```python
from build123d import *

# Parameters (mm, degrees)
BOSS_EXTRUDE1_DEPTH = 3.175
SKETCH3_R           = 1.47
CUT_EXTRUDE5_DEPTH  = 10
CUT_EXTRUDE6_DEPTH  = 10
BOSS_EXTRUDE2_DEPTH = 3.175
SKETCH7_R           = 1.5
CUT_EXTRUDE7_DEPTH  = 10
SKETCH9_R           = 1.5
CUT_EXTRUDE9_DEPTH  = 10
CUT_EXTRUDE10_DEPTH = 10
SKETCH11_R          = 1.5
CUT_EXTRUDE11_DEPTH = 10


with BuildPart() as part:
    # Sketch1 → Boss-Extrude1 (new body)
    with BuildSketch(Plane.XY):
        Polygon((-26.794919243, 100), (26.794919243, 100), (73.205080757, 73.205080757), (100, 26.794919243), (100, -26.794919243), (73.205080757, -73.205080757), (26.794919243, -100), (-26.794919243, -100), (-73.205080757, -73.205080757), (-100, -26.794919243), (-100, 26.794919243), (-73.205080757, 73.205080757), align=None)
    extrude(amount=BOSS_EXTRUDE1_DEPTH)

    # Sketch3 → Cut-Extrude5 (cut)
    with BuildSketch(Plane(origin=(0, 0, 0), x_dir=(-1, 0, 0), z_dir=(0, 0, -1))):
        Polygon((51.443588913, -82.102909721), (53.031088913, -84.852540378), (73.205080757, -73.205080757), (84.852540378, -53.031088913), (82.102909721, -51.443588913), (70.880819443, -70.880819443), align=None)
        Polygon((-26.794919243, -100), (-3.5, -100), (-3.5, -96.825), (-25.944180557, -96.825), (-45.381411087, -85.602909721), (-46.968911087, -88.352540378), align=None)
        Polygon((-73.205080757, -73.205080757), (-53.031088913, -84.852540378), (-51.443588913, -82.102909721), (-70.880819443, -70.880819443), (-82.102909721, -51.443588913), (-84.852540378, -53.031088913), align=None)
        with Locations((-49.20625, -85.22772505)):
            Circle(SKETCH3_R)
        Polygon((-100, -26.794919243), (-88.352540378, -46.968911087), (-85.602909721, -45.381411087), (-96.825, -25.944180557), (-96.825, -3.5), (-100, -3.5), align=None)
        Polygon((-100, 26.794919243), (-100, 3.5), (-96.825, 3.5), (-96.825, 25.944180557), (-85.602909721, 45.381411087), (-88.352540378, 46.968911087), align=None)
        Polygon((-26.794919243, 100), (-46.968911087, 88.352540378), (-45.381411087, 85.602909721), (-25.944180557, 96.825), (-3.5, 96.825), (-3.5, 100), align=None)
        Polygon((26.794919243, 100), (3.5, 100), (3.5, 96.825), (25.944180557, 96.825), (45.381411087, 85.602909721), (46.968911087, 88.352540378), align=None)
        Polygon((73.205080757, 73.205080757), (53.031088913, 84.852540378), (51.443588913, 82.102909721), (70.880819443, 70.880819443), (82.102909721, 51.443588913), (84.852540378, 53.031088913), align=None)
        with Locations((-85.22772505, 49.20625)):
            Circle(SKETCH3_R)
        with Locations((-49.20625, 85.22772505)):
            Circle(SKETCH3_R)
        with Locations((0, 98.4125)):
            Circle(SKETCH3_R)
        with Locations((49.20625, 85.22772505)):
            Circle(SKETCH3_R)
        with Locations((85.22772505, 49.20625)):
            Circle(SKETCH3_R)
        with Locations((98.4125, 0)):
            Circle(SKETCH3_R)
        Polygon((96.825, -3.5), (96.825, -25.944180557), (85.602909721, -45.381411087), (88.352540378, -46.968911087), (100, -26.794919243), (100, -3.5), align=None)
        with Locations((85.22772505, -49.20625)):
            Circle(SKETCH3_R)
        Polygon((45.381411087, -85.602909721), (25.944180557, -96.825), (3.5, -96.825), (3.5, -100), (26.794919243, -100), (46.968911087, -88.352540378), align=None)
        with Locations((0, -98.4125)):
            Circle(SKETCH3_R)
        with Locations((49.20625, -85.22772505)):
            Circle(SKETCH3_R)
        with Locations((-85.22772505, -49.20625)):
            Circle(SKETCH3_R)
        with Locations((-98.4125, 0)):
            Circle(SKETCH3_R)
        Polygon((-82.102909721, 51.443588913), (-70.880819443, 70.880819443), (-51.443588913, 82.102909721), (-53.031088913, 84.852540378), (-73.205080757, 73.205080757), (-84.852540378, 53.031088913), align=None)
        Polygon((100, 26.794919243), (88.352540378, 46.968911087), (85.602909721, 45.381411087), (96.825, 25.944180557), (96.825, 3.5), (100, 3.5), align=None)
    extrude(amount=-CUT_EXTRUDE5_DEPTH, mode=Mode.SUBTRACT)

    # Sketch4 → Cut-Extrude6 (cut)
    with BuildSketch(Plane.XY.offset(3.175)):
        Polygon((27.531680557, 99.574630657), (25.944180557, 96.825), (96.825, -25.944180557), (100, -25.944180557), (100, 27.816263625), (73.190593106, 73.213445206), align=None)
    extrude(amount=-CUT_EXTRUDE6_DEPTH, mode=Mode.SUBTRACT)

    # Sketch5 → Boss-Extrude2 (add)
    with BuildSketch(Plane.XY.offset(3.175)):
        Polygon((96.825, -25.944180557), (143.278603525, 0.875819943), (72.397784082, 123.6450005), (25.944180557, 96.825), align=None)
    extrude(amount=-BOSS_EXTRUDE2_DEPTH)

    # Sketch7 → Cut-Extrude7 (cut)
    with BuildSketch(Plane(origin=(0, 0, 0), x_dir=(-1, 0, 0), z_dir=(0, 0, -1))):
        with Locations((-119.051801763, -10.8021295)):
            Circle(SKETCH7_R)
        with Locations((-50.17098232, 108.502949442)):
            Circle(SKETCH7_R)
    extrude(amount=-CUT_EXTRUDE7_DEPTH, mode=Mode.SUBTRACT)

    # Sketch9 → Cut-Extrude9 (cut)
    with BuildSketch(Plane(origin=(0, 0, 0), x_dir=(-1, 0, 0), z_dir=(0, 0, -1))):
        with Locations((73.306739868, -14.507270856)):
            Circle(SKETCH9_R)
        with Locations((21.70291705, -2.187552088)):
            Circle(SKETCH9_R)
        with Locations((7.673469234, -26.303617148)):
            Circle(SKETCH9_R)
    extrude(amount=-CUT_EXTRUDE9_DEPTH, mode=Mode.SUBTRACT)

    # Sketch10 → Cut-Extrude10 (cut)
    with BuildSketch(Plane.XY.offset(3.175)):
        Polygon((27.153871113, -53.276548933), (85.191651102, -19.768396257), (26.553283992, 81.796259373), (-31.484495997, 48.288106697), align=None)
    extrude(amount=-CUT_EXTRUDE10_DEPTH, mode=Mode.SUBTRACT)

    # Sketch11 → Cut-Extrude11 (cut)
    with BuildSketch(Plane.XY.offset(3.175)):
        with Locations((64.18037908, -50.392061509)):
            Circle(SKETCH11_R)
        with Locations((-9.45962092, 77.156159961)):
            Circle(SKETCH11_R)
    extrude(amount=-CUT_EXTRUDE11_DEPTH, mode=Mode.SUBTRACT)


solid = part.part
```
Input: part model. Units: mm. Frame: model coordinates. A direction names the side the tool comes from. Coordinates: 2 decimals unless noted, no trailing zeros. Loops run counter-clockwise (first coordinate to the right, second up) from the corner with the lowest first, then second, coordinate; pieces in that order, holes last.
Q1. Line query: line 1 along Y through (x, z) = (-52.5, 1.7); line 2 along X through (y, z) = (-84, 2.65); line 3 along Y through (x, z) = (52.5, 2.05). Output: solid intervals per line, ascending.
Results are:
line 1: y = -85.16 to -83.93, -81.49 to 81.49, 83.93 to 85.16
line 2: x = -52.54 to -50.01, -48.4 to 48.4, 50.01 to 52.54
line 3: y = -85.16 to -83.93, -81.49 to -38.64, 36.86 to 112.16
Q2. Section D-D, the plane y = -66. Return the cut outline in (x, z) (3 decimals), and give its area (3 significant figures).
Results are:
outline: (-73.699, 0) - (73.699, 0) - (73.699, 3.175) - (-73.699, 3.175) - close
area: 468 mm2
Q3. Contact query for flat-ended pins moving along their axis: pin 1 (1.6 mm diameter, centred on y = -17, z = 2, fed in from -X) (3 decimals); pin 2 (1 mm diameter, centred on x = -21.5, z = 2.5, fed in from -Y) (3 decimals); pin 3 (1 mm diameter, centred on y = 35, z = 1.5, fed in from -X); pin 4 (4.5 mm diameter, centred on x = 85.23, y = -49.21, fed in from +Z) (3 decimals). Output: stop coordinate, or through.
Results are:
pin 1: stops at x = -96.825
pin 2: stops at y = -96.825
pin 3: stops at x = -91.89
pin 4: stops at z = 3.175
Q4. Section C-C, the plane z = 0.65. Give the number of separate pieces and of enclosed holes in the cut face, and give its area (3 significant figures).
Results are:
separate pieces: 1
enclosed holes: 17
area: 27,500 mm2
Q5. Section B-B, the plane x = 8. Return the cut outline in (y, z) (1 decimal), and give its area (3 significant figures).
Results are:
outline: (-96.8, 0) - (-20.1, 0) - (-20.1, 3.2) - (-96.8, 3.2) - close; (71.1, 0) - (96.8, 0) - (96.8, 3.2) - (71.1, 3.2) - close
area: 325 mm2
Q6. Mould query, pull axis X, two halves, no side actions, for faces 1 (the flat face through (-35.799, -91.135, 1.565)), 2 (the flat face through (55.766, -36.757, 1.61)), 3 (the flat face through (108.334, 61.401, 1.61)), 4 (the flat face through (-61.03, 76.57, 1.57)). Classes: +X half, -X half, draft (parallel to the pull), parting line (faces both ways), or undercut.
Results are:
face 1: undercut
face 2: undercut
face 3: +X half
face 4: -X half
Q7. Section A-A, the plane y = 41.5. Return the cut outline in (x, z) (3 decimals), and give its area (3 significant figures).
Results are:
outline: (-87.844, 0) - (-27.565, 0) - (-27.565, 3.175) - (-87.844, 3.175) - close; (49.818, 0) - (119.824, 0) - (119.824, 3.175) - (49.818, 3.175) - close
area: 414 mm2
Q8. Set-up query: faces 5 (the flat face through (-91.135, 35.799, 1.565)), 6 (the flat face through (-2.059, 65.277, 1.61)), 7 (the flat face through (-35.53, 91.29, 1.57)), 8 (the flat face through (91.135, -35.799, 1.565)). Return all of +Z, -Z, +X, -X, +Y, -Y with unobstructed straight access to the full face (end or side cutting, diameter ignored); none if empty.
Results are:
face 5: +Z, -Z, -X
face 6: +Z, -Z
face 7: +Z, -Z, +Y
face 8: +Z, -Z, +X
